Could you check a few things on this drawing? It's one solid part, dimensions in mm from its lowest x, y, z. Give positions to 0.01 mm unless a question says otherwise; leave off trailing zeros. Order: outer loops, then holes, each group sorted by start corner. A loop starts at its lowest first (then second) coordinate and runs counter-clockwise, first axis right, second up. Notation, with made-up numbers: (87.25, -29) -> (95.25, -29) arc R21 ccw to (95.25, -21) -> close; hole circle Ø3 at (-31, -4). An arc over 180 degrees is marked (long way). Write each question's results on one line, items separated by ' | '. Start each with the question number.
Q1. Imagine slicing it at A-A, the plane y = 22.2. Please give me the cut outline in (x, z).
Q2. Imagine slicing it at D-D, the plane z = 30. Please give me the cut outline in (x, y), then the cut area to 3 significant figures.
Q3. Imagine slicing it at C-C, the plane x = 22.7. Please give me the cut outline in (y, z), then the cut area to 3 significant figures.
Q4. I'm going to push flat-ended pins straight in: pin 1 (4 mm diameter, centred on x = 18.5, y = 5, fed in from -Z); pin 2 (1 mm diameter, centred on y = 8, z = 16.5, fed in from +X); pin 3 (1 mm diameter, centred on y = 37, z = 34.5, fed in from +X); pin 4 (1.5 mm diameter, centred on x = 12, z = 51.5, fed in from -Y). Where does each tip first touch, or does it pass through?
Q5. I need wall thicknesses on line 1 along Y through (x, z) = (22, 24); line 2 along Z through (x, y) = (22.7, 44.1). Which ranges of each line are inside material? Lowest first, please. Write a range as [from, to].
Q6. Imagine slicing it at B-B, the plane x = 30. Please give me the cut outline in (y, z).
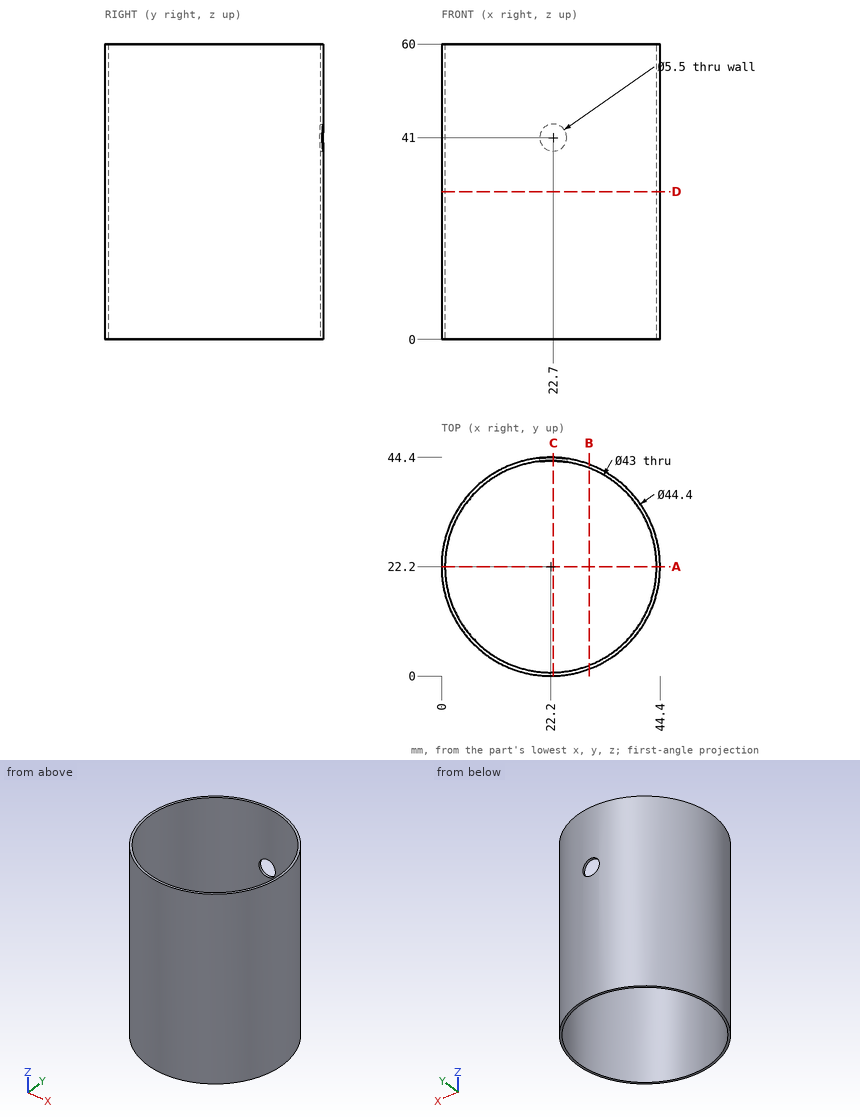
Geometry check:
1) outline: (0, 0) -> (0.7, 0) -> (0.7, 60) -> (0, 60) -> close; (43.7, 0) -> (44.4, 0) -> (44.4, 60) -> (43.7, 60) -> close
2) outline: circle Ø44.4 at (22.2, 22.2); hole circle Ø43 at (22.2, 22.2) | area: 96.1 mm²
3) outline: (0.01, 0) -> (0.71, 0) -> (0.71, 60) -> (0.01, 60) -> close; (43.69, 0) -> (44.39, 0) -> (44.39, 38.25) -> (43.69, 38.25) -> close; (43.69, 43.75) -> (44.39, 43.75) -> (44.39, 60) -> (43.69, 60) -> close | area: 80.2 mm²
4) pin 1: through | pin 2: x = 39.67 | pin 3: x = 39.18 | pin 4: y = 2.11
5) line 1: [0, 0.7], [43.7, 44.4] | line 2: [0, 38.25], [43.75, 60]
6) outline: (1.42, 0) -> (2.16, 0) -> (2.16, 60) -> (1.42, 60) -> close; (42.24, 0) -> (42.98, 0) -> (42.98, 60) -> (42.24, 60) -> close
